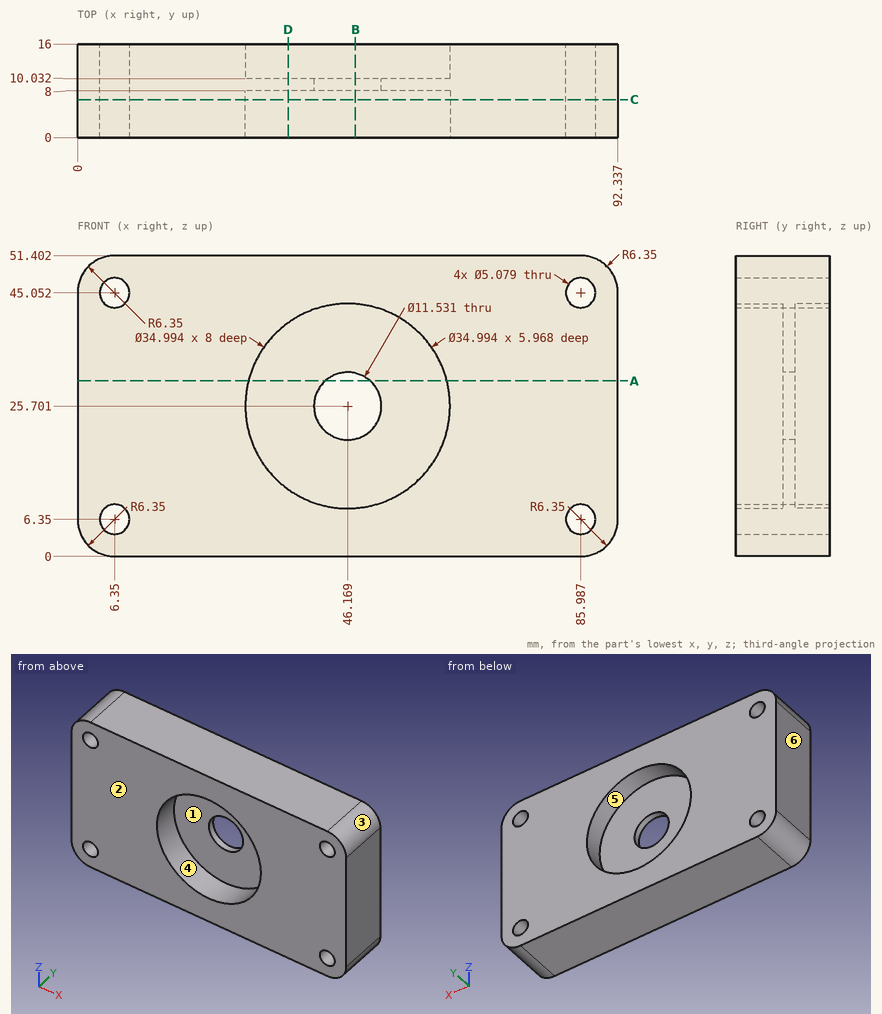
Geometry check sheet. Reference: drawing and pictorial views, mm from the part's lowest x, y, z. A direction names the side the tool comes from. Give positions to 0.01 mm unless a question says otherwise; leave off trailing zeros. Order: outer loops, then holes, each group sorted by start corner. A loop starts at its lowest first (then second) coordinate and runs counter-clockwise, first axis right, second up. Notation, with made-up numbers: M 86,16.5 L 106,16.5 A27 cw 106,48.5 Z; hole C 84.5,-18.75 d6. An arc over 180 degrees is marked long. Answer as CSV lines item,"result". Start each with the question number.
Item 1: Cross-section at C-C on y = 6.5. State how many separate pieces and enclosed holes the cut face has, plus the area to 3 significant figures.
Item 2: Tool access check on the marked faces 4, 5 and 6. Record the directions out of +Z, -Z, +X, -X, +Y, -Y that give a thin tool (end or side, any length) a straight path to the whole face; none if there is none.
Item 3: Cross-section at A-A on z = 30. Enter the section's corners in (x, y), plus the area to 3 significant figures.
Item 4: Mould release check, pull along X, two halves, no side actions. Record for the marked faces 1, 2 and 3: +X half, -X half, draft (parallel to the pull), parting line (faces both ways), or undercut.
Item 5: Cross-section at B-B on x = 47.5. Enter the section's corners in (y, z) (1 decimal), plus the area to 3 significant figures.
Item 6: Cross-section at D-D on x = 36. Enter the section's corners in (y, z).
Item 7: Gauge pin test, flat ends, axial feed: P1, Ø3, axis at x = 67, z = 37, coming from the -Y side; P2, Ø10.5, axis at x = 45.5, z = 26, coming from the +Y side; P3, Ø10.5, axis at x = 53.5, z = 28.5, coming from the -Y side; P4, Ø4.5, axis at x = 85.99, z = 45.05, coming from the +Y side. Record the tip position at first contact, or that the pin passes through.
Item 8: Thickness scan on line 1 (Z direction, x = 45.5, y = 5.25) (1 decimal); line 2 (X direction, y = 10, z = 7) (1 decimal); line 3 (X direction, y = 3, z = 47) (1 decimal). Record the ranges inside material, lowest first. Write a range as [from, to].
Established:
1,separate pieces,"1"
1,enclosed holes,"5"
1,area,"3,670 mm^2"
2,face 4,"-Y"
2,face 5,"+Y"
2,face 6,"+Z, -Z, -X, +Y, -Y"
3,outline,"M 0,0 L 29.21,0 L 29.21,8 L 42.33,8 L 42.33,10.03 L 29.21,10.03 L 29.21,16 L 0,16 Z; M 50.01,8 L 63.13,8 L 63.13,0 L 92.34,0 L 92.34,16 L 63.13,16 L 63.13,10.03 L 50.01,10.03 Z"
3,area,"988 mm^2"
4,face 1,"undercut"
4,face 2,"draft"
4,face 3,"+X half"
5,outline,"M 0,0 L 16,0 L 16,8.3 L 10,8.3 L 10,20.1 L 8,20.1 L 8,8.3 L 0,8.3 Z; M 0,43.1 L 8,43.1 L 8,31.3 L 10,31.3 L 10,43.1 L 16,43.1 L 16,51.4 L 0,51.4 Z"
5,area,"312 mm^2"
6,outline,"M 0,0 L 16,0 L 16,11.46 L 10.03,11.46 L 10.03,39.94 L 16,39.94 L 16,51.4 L 0,51.4 L 0,39.94 L 8,39.94 L 8,11.46 L 0,11.46 Z"
7,P1,"stops at y = 0"
7,P2,"stops at y = 10.03"
7,P3,"stops at y = 8"
7,P4,"passes through"
8,line 1,"z = [0, 8.2], [43.2, 51.4]"
8,line 2,"x = [0, 3.9], [8.8, 83.5], [88.4, 92.3]"
8,line 3,"x = [0.3, 4.7], [8, 84.4], [87.6, 92]"
